Check sheet for the modelled part. Datum: model origin and axes. Units: mm. A direction names the side the tool comes from. Coordinates: 2 decimals unless noted, no trailing zeros. Loops run counter-clockwise (first coordinate to the right, second up) from the corner with the lowest first, then second, coordinate; pieces in that order, holes last. Notation, with made-up numbers: (46, -34.5) -> (53, -34.5) arc R26 cw to (53, -4.5) -> close; hole circle Ø2 at (1.25, 59). An arc over 180 degrees is marked (long way). Use one line per item in the form item = value.
from build123d import *

# Parameters (mm, degrees)
SKETCH1_W           = 50
SKETCH1_H           = 10
BOSS_EXTRUDE1_DEPTH = 5
SKETCH2_R           = 2.5
SKETCH2_R_2         = 2
CUT_EXTRUDE1_DEPTH  = 5
SKETCH3_R           = 2
CUT_EXTRUDE2_DEPTH  = 5
CUT_EXTRUDE3_DEPTH  = 2
SKETCH5_R           = 2.5
BOSS_EXTRUDE2_DEPTH = 2
FILLET1_R           = 1


with BuildPart() as part:
    # Sketch1 → Boss-Extrude1 (new body)
    with BuildSketch(Plane(origin=(0, 0, 0), x_dir=(1, 0, 0), z_dir=(0, 1, 0))):
        with Locations((25, 5)):
            Rectangle(SKETCH1_W, SKETCH1_H)
    extrude(amount=BOSS_EXTRUDE1_DEPTH)

    # Sketch2 → Cut-Extrude1 (cut)
    with BuildSketch(Plane.XZ):
        with Locations(Location((5, -5, 0), (0, 0, 270))):
            Circle(SKETCH2_R)
        with Locations(Location((11.5, -5, 0), (0, 0, 270))):
            Circle(SKETCH2_R_2)
    extrude(amount=-CUT_EXTRUDE1_DEPTH, mode=Mode.SUBTRACT)

    # Sketch3 → Cut-Extrude2 (cut)
    with BuildSketch(Plane(origin=(0, 5, 0), x_dir=(1, 0, 0), z_dir=(0, 1, 0))):
        with Locations(Location((35, 5, 0), (0, 0, 270))):
            Circle(SKETCH3_R)
    extrude(amount=-CUT_EXTRUDE2_DEPTH, mode=Mode.SUBTRACT)

    # Sketch4 → Cut-Extrude3 (cut)
    with BuildSketch(Plane(origin=(0, 5, 0), x_dir=(1, 0, 0), z_dir=(0, 1, 0))):
        Polygon((11.5, 0.8), (15.137306696, 2.9), (15.137306696, 7.1), (11.5, 9.2), (7.862693304, 7.1), (7.862693304, 2.9), align=None)
    extrude(amount=-CUT_EXTRUDE3_DEPTH, mode=Mode.SUBTRACT)

    # Sketch5 → Boss-Extrude2 (add)
    with BuildSketch(Plane(origin=(0, 5, 0), x_dir=(1, 0, 0), z_dir=(0, 1, 0))):
        with Locations(Location((41.5, 5, 0), (0, 0, 90))):
            Circle(SKETCH5_R)
    extrude(amount=BOSS_EXTRUDE2_DEPTH)

    # Fillet1
    fillet1_edges = [part.edges().sort_by_distance(p)[0] for p in [
        (41.5, 7, -2.5),
    ]]
    fillet(fillet1_edges, radius=FILLET1_R)

    # Boss-Extrude3 cone 1 section (through the dimple's axis) → Boss-Extrude3 (revolve)
    with BuildSketch(Plane(origin=(50, 2.5, -5), x_dir=(0, 0, 1), z_dir=(0, 1, 0))):
        Polygon((0, 0), (2.5, 0), (0, 7.694208843), align=None)
    revolve(axis=Axis((50, 2.5, -5), (1, 0, 0)))


solid = part.part
(1) Mould release check, pull along Z, two halves, no side actions. Record for faces 4 (the flat face through (25, 2, -10)), 5 (the cylindrical face through (12.852, 1.479, -3.526)), 6 (the flat face through (50, 2, -1)): +Z half, -Z half, draft (parallel to the pull), parting line (faces both ways), or undercut.
Established:
face_4 = -Z half
face_5 = undercut
face_6 = draft
(2) Go/stop test with flat-tipped pins: P1, Ø5, axis at x = 13, z = -1.5, coming from the +Y side; P2, Ø3.5, axis at x = 35, z = -5, coming from the -Y side. Record where each tip stops, or that it passes through.
Established:
P1 = 5
P2 = through
(3) Section check B-B, the plane x = 41.5. Record the boundary of the cut face in (y, z), plus the area to 3 significant figures.
Established:
outline = (0, -10) -> (5, -10) -> (5, -7.5) -> (6, -7.5) arc R1 ccw to (7, -6.5) -> (7, -3.5) arc R1 ccw to (6, -2.5) -> (5, -2.5) -> (5, 0) -> (0, 0) -> close
area = 59.6 mm²
(4) Section check A-A, the plane x = 35. Record the boundary of the cut face in (y, z).
Established:
outline = (0, -10) -> (5, -10) -> (5, -7) -> (0, -7) -> close; (0, -3) -> (5, -3) -> (5, 0) -> (0, 0) -> close
(5) Tool access check on faces 1 (the flat face through (0, 2, -5)), 2 (the flat face through (9.656, 4.014, -1.865)), 3 (the flat face through (50, 2, -9)). Record the directions out of +Z, -Z, +X, -X, +Y, -Y that give a thin tool (end or side, any length) a straight path to the whole face; none if there is none.
Established:
face_1 = +Z, -Z, -X, +Y, -Y
face_2 = +Y
face_3 = -Z, +X
(6) Section check C-C, the plane y = 4. Give the number of separate pieces and of enclosed holes in the cut face, plus the area to 3 significant figures.
Established:
separate_pieces = 1
enclosed_holes = 3
area = 430 mm²
(7) Scan lines: line 1 along X through (y, z) = (0.75, -6.75); line 2 along Y through (x, z) = (12, -1); line 3 along Z through (x, y) = (10.5, 4). Record each from-to range of solid material in increasing order.
Established:
line_1 = 0 to 3.21, 6.79 to 10.53, 12.47 to 34.03, 35.97 to 50.08
line_2 = 0 to 5
line_3 = -10 to -8.62, -1.38 to 0
